from build123d import *

# Parameters (mm, degrees)
BOSS_EXTRUDE1_DEPTH = 75
SKETCH2_W           = 33.479779341
SKETCH2_H           = 3
BOSS_EXTRUDE2_DEPTH = 9


with BuildPart() as part:
    # Sketch1 → Boss-Extrude1 (new body)
    with BuildSketch(Plane.XY):
        with BuildLine():
            Line((11.575975539, 13.62181128), (13.040589352, 11.003623667))
            Line((13.040589352, 11.003623667), (2.567838899, 5.145168413))
            Line((2.567838899, 5.145168413), (4.032452713, 2.5269808))
            Line((4.032452713, 2.5269808), (24.602620365, 14.033929934))
            ThreePointArc((24.602620365, 14.033929934), (26.034093135, 14.56730426), (27.559801463, 14.643570636))
            Line((27.559801463, 14.643570636), (60.860709888, 11.187398941))
            Line((60.860709888, 11.187398941), (61.170404733, 14.171370975))
            Line((61.170404733, 14.171370975), (49.231357904, 15.379328261))
            Line((49.231357904, 15.379328261), (49.533347225, 18.364089968))
            Line((49.533347225, 18.364089968), (26.242046455, 20.781403438))
            ThreePointArc((26.242046455, 20.781403438), (24.716338127, 20.705137062), (23.284865357, 20.171762736))
            Line((23.284865357, 20.171762736), (11.575975539, 13.62181128))
        make_face()
    extrude(amount=BOSS_EXTRUDE1_DEPTH)

    # Sketch2 → Boss-Extrude2 (add)
    with BuildSketch(Plane(origin=(1.797301431, 17.317360261, 0), x_dir=(0.9946573448357569, -0.10323161513936713, 0), z_dir=(-0.10323161513936711, -0.9946573448357567, 0))):
        with Locations((42.64076917, 73.5)):
            Rectangle(SKETCH2_W, SKETCH2_H)
    extrude(amount=BOSS_EXTRUDE2_DEPTH)


solid = part.part
Read the model definition and answer for the solid it produces. Units are mm, in the model's axes. A direction names the side the tool comes from. Round coordinates to 2 decimals unless told otherwise and drop trailing zeros. Write each loop counter-clockwise with the first axis right and the second up, starting at its lowest first coordinate (ties: lowest second). Pieces come first, ordered by that corner, then holes. Notation, with made-up numbers: (70.5, 52) - (92.5, 52) arc R30 cw to (92.5, 79) - close; hole circle Ø1 at (-4.75, 34). An arc over 180 degrees is marked (long way). Use a Markdown table: item, result.
(1) The part is cut by section A-A (y = 9). Write down the section's boundary in (x, z).
Reported:
| item | result |
|---|---|
| outline | (9.46, 0) - (15.6, 0) - (15.6, 75) - (9.46, 75) - close; (26.97, 72) - (60.63, 72) - (60.63, 75) - (26.97, 75) - close |
(2) Each of these flat-tipped pins is pushed along its axis until it touches: pin 1 Ø6 at (x, y) = (44, 11) entering from -Z; pin 2 Ø1 at (x, y) = (33, 6) entering from -Z; pin 3 Ø2 at (x, z) = (45, 57) entering from -Y; pin 4 Ø10 at (x, z) = (38.5, 17.5) entering from +Y. Where does it stop, or does it pass through?
Reported:
| item | result |
|---|---|
| pin 1 | z = 0 |
| pin 2 | z = 72 |
| pin 3 | y = 12.73 |
| pin 4 | y = 20.03 |
(3) Straight lines are drawn through the part: line 1 along Z through (x, y) = (44.5, 12.5); line 2 along Y through (x, z) = (45.5, 68); line 3 along X through (y, z) = (4, 43.5). For each, find the intervals that lie inside material, in ascending order. Write a range as [from, to].
Reported:
| item | result |
|---|---|
| line 1 | [72, 75] |
| line 2 | [12.78, 18.78] |
| line 3 | [3.21, 6.67] |
(4) The part is cut by section C-C (x = 33). Write down the section's boundary in (y, z).
Reported:
| item | result |
|---|---|
| outline | (5.03, 72) - (14.08, 72) - (14.08, 0) - (20.08, 0) - (20.08, 75) - (5.03, 75) - close |
(5) The mould has two halves that part along Y. Classify faces 1 (the flat face through (43.048, 3.988, 73.521)), 2 (the flat face through (27.1, 10.2, 73.5)), 3 (the flat face through (12.3, 12.33, 36.98)), 4 (the cylindrical face through (24.7, 20.7, 37)): released by +Y, released by -Y, zero draft, split by the parting line, or undercut.
Reported:
| item | result |
|---|---|
| face 1 | released by -Y |
| face 2 | undercut |
| face 3 | undercut |
| face 4 | released by +Y |
(6) The part is cut by section B-B (z = 9.5). Write down the section's boundary in (x, y), then the cut area to 3 significant figures.
Reported:
| item | result |
|---|---|
| outline | (2.57, 5.15) - (4.03, 2.53) - (24.6, 14.03) arc R5 cw to (27.56, 14.64) - (60.86, 11.19) - (61.17, 14.17) - (49.23, 15.38) - (49.53, 18.36) - (26.24, 20.78) arc R5 ccw to (23.28, 20.17) - (11.58, 13.62) - (13.04, 11) - close |
| area | 300 mm2 |
(7) The part is cut by section D-D (x = 9.5). Write down the section's boundary in (y, z), then the cut area to 3 significant figures.
Reported:
| item | result |
|---|---|
| outline | (5.59, 0) - (9.02, 0) - (9.02, 75) - (5.59, 75) - close |
| area | 258 mm2 |
(8) Which of the six approach directions +Z, -Z, +X, -X, +Y, -Y give full straight-line access (tool end or side, diameter ignored) to faces 5 (the flat face through (17.51, 16.94, 36.98)), 6 (the flat face through (44, 9, 72)), 7 (the flat face through (14.17, 8.2, 36.98)), 8 (the flat face through (49.38, 16.85, 36.98))?
Reported:
| item | result |
|---|---|
| face 5 | +Z, -Z, -X, +Y |
| face 6 | -Z, -Y |
| face 7 | +Z, -Z, -Y |
| face 8 | +Z, -Z, +X |
